Part model, mm, in its own coordinate system. A direction names the side the tool comes from. Round coordinates to 2 decimals unless told otherwise and drop trailing zeros. Loops run counter-clockwise (first coordinate to the right, second up) from the corner with the lowest first, then second, coordinate; pieces in that order, holes last. Notation, with made-up numbers: (-26.75, 23.5) -> (-10.75, 23.5) arc R15 ccw to (-10.75, 51.5) -> close; hole circle Ø1 at (11.25, -30). An arc over 180 degrees is marked (long way). Answer as CSV lines item,"result".
from build123d import *

# Parameters (mm, degrees)
F0_R     = 4
F1_DEPTH = 3.5
F2_R     = 6
F3_DEPTH = 1
F4_R     = 11
F5_DEPTH = 1
F6_SIZE  = 0.99999
F8_DEPTH = 0.3


# Not quite as in the source:
# - a fillet or chamfer is up to 0.001 mm smaller than in the source, because OpenCascade refuses the exact size


with BuildPart() as f1:
    # F0 (on Top) → F1 (new body)
    with BuildSketch(Plane.XY):
        Circle(F0_R)
    extrude(amount=F1_DEPTH)

    # F2 (on face) → F3 (join)
    with BuildSketch(Plane.XY.offset(3.5)):
        Circle(F2_R)
    extrude(amount=F3_DEPTH)

    # F4 (on face) → F5 (join)
    with BuildSketch(Plane.XY.offset(4.5)):
        Circle(F4_R)
    extrude(amount=F5_DEPTH)

    # F6 (size 1 in the source; OpenCascade refuses exactly that, so slightly less here)
    f6_edges = [f1.edges().sort_by_distance(p)[0] for p in [
        (-11, 0, 5.5),
    ]]
    chamfer(f6_edges, length=F6_SIZE)

    # F7 (on face) → F8 (cut)
    with BuildSketch(Plane.XY.offset(5.5)):
        Polygon((1.3699667839, 6.4073562332), (-0.3065554774, 2.496608533), (-7.2352840317, -2.3525079081), (-7.2352840317, -4.5790599288), (-2.2722620734, -1.0865629438), (-2.2722620734, -4.7009375549), (-2.7038290382, -5.1864506813), (-2.7038290382, -6.4811520415), (0.2092490221, -4.7009375549), (0.2092490221, -3.5950467127), (-0.3302100332, -3.8378033924), (-0.57296648, -0.6819687688), (1.099356149, -3.1634797479), (2.4749761405, -3.1634797479), (3.8502510524, -3.1634797479), (3.8502510524, 4.6872763105), (3.8502510524, 6.4073562332), align=None)
    extrude(amount=-F8_DEPTH, mode=Mode.SUBTRACT)


solid = f1.part
Q1. Which spindle directions (+Z, -Z, +X, -X, +Y, -Y) get a long thin tool onto all of the face, cutting with end or side? Do faces 5 (the face through (0, -2, 5.5)), 6 (the face through (5, -5, 4.5)). Say none if no direction does.
Geometry results:
face 5,"+Z, +X, -X, +Y, -Y"
face 6,"-Z"
Q2. Saw through at B-B, the plane z = 1. Write the cut outline in (x, y), then the cut area to 3 significant figures.
Geometry results:
outline,"circle Ø8 at (0, 0)"
area,"50.3 mm2"
Q3. Two-plate mould, pull along Y, no slides. Class faces 1 (the face through (0, 0, 0)), 2 (the face through (-4.79, -2.86, 5.35)), 3 (the face through (-3.72, 0.11, 5.35)), 4 (the face through (-0.867, -3.905, 1.726)): pulls with the +Y half, pulls with the -Y half, needs draft (parallel to the pull), parting line crosses it, or undercut.
Geometry results:
face 1,"needs draft"
face 2,"undercut"
face 3,"undercut"
face 4,"parting line crosses it"
Q4. Drill centre lines: line 1 along Z through (x, y) = (1.5, -1); line 2 along Z through (x, y) = (4.75, 3.75); line 3 along Y through (x, z) = (-0.25, 3.2). Where is each one in solid material? Low to high.
Geometry results:
line 1,"0 to 5.2"
line 2,"4.5 to 5.5"
line 3,"-3.99 to 3.99"
Q5. Drop flat-ended pins along their axis: P1, Ø12, axis at x = -3, y = 0.5, coming from the +Z side; P2, Ø1.5, axis at y = -1.5, z = 3, coming from the -X side; P3, Ø2, axis at x = -4, y = -4.5, coming from the -Z side; P4, Ø3, axis at y = 8.5, z = 2, coming from the +X side (3 decimals). Give the stop position or say it passes through.
Geometry results:
P1,"z = 5.5"
P2,"x = -5.93"
P3,"z = 3.5"
P4,"through"
